Can you work these out from the model? Positions are in its coordinate system, mm. Face numbers are marked on the shaded views. Round coordinates to 2 decimals unless told otherwise and drop trailing zeros. Write each loop counter-clockwise with the first axis right and the second up, starting at its lowest first coordinate (ties: lowest second). Pieces come first, ordered by that corner, then holes. Notation, with made-up numbers: M 69.5,39 L 83.5,39 A6 ccw 83.5,50 Z; hole C 13,89 d5. An arc over 180 degrees is marked long. Answer in a Markdown table with one row per item. Add a question column.
(1) Suppose I cut it at A-A, the plane y = -40. Write out the boundary of the cut face in (x, z).
(2) I'm going to push flat-ended pins straight in: pin 1 (3.5 mm diameter, centred on x = -180.65, z = 32.92, fed in from +Y); pin 2 (12 mm diameter, centred on x = -61.5, y = 3.5, fed in from +Z); pin 3 (1 mm diameter, centred on x = -120.5, z = -0.5, fed in from -Y); pin 4 (1 mm diameter, centred on x = -169, z = 8, fed in from -Y). Where does each tip first touch, or does it pass through?
(3) If I drill on probe 1 along X at (y, z) = (-35, -1); probe 2 along X at (y, z) = (-50, -0.4); probe 3 along X at (y, z) = (76, 12), over which ranges is the centre line in solid material (lowest first)?
(4) Suppose I cut it at C-C, the plane z = 12.5. Write out the boundary of the cut face in (x, y), then the cut area to 3 significant figures.
(5) Suppose I cut it at B-B, the plane x = -92. Write out the boundary of the cut face in (y, z).
(6) If we mould it in two halves opening along Y, with no side actions, what happens to the marked faces 1 and 2? For each: released by +Y, released by -Y, zero draft, split by the parting line, or undercut.
(7) Suppose I cut it at D-D, the plane y = -15.5. Write out the boundary of the cut face in (x, z), then the cut area to 3 significant figures.
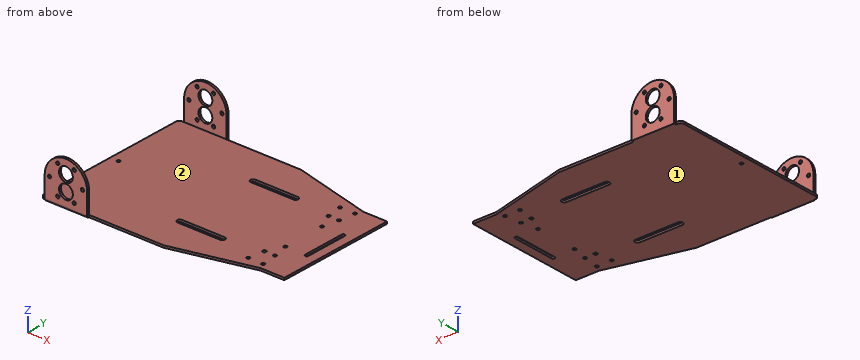
Autodesk Inventor part; units mm, degrees
ref_plane "YZ Plane" through (0, 0, 0) normal (1, 0, 0) x (0, 1, 0)
ref_plane "XZ Plane" through (0, 0, 0) normal (0, 1, 0) x (-1, 0, 0)
ref_plane "XY Plane" through (0, 0, 0) normal (0, 0, 1) x (1, 0, 0)
ref_plane "Plano de trabajo1" through (0, 0, 0) normal (0, 0, 1) x (1, 0, 0)
sketch "Boceto1" plane through (0, 0, 0) normal (0, 0, 1) x (1, 0, 0)
  line L0 (14.1, -53) -> (14.1, 53)
  line L1 (-197.9, 72) -> (-197.9, -72)
  line L2 (-194.9, -75) -> (-82.9, -75)
  line L3 (-7.9, -56) -> (14.1, -56)
  line L4 (5.6, 20) -> (5.6, -20)
  line L5 (2.6, -20) -> (2.6, 20)
  circle A0 centre (4.1, -20) radius 1.5
  circle A1 centre (4.1, 20) radius 1.5
  line L6 (-14.4, 20) -> (-14.4, -20)
  line L7 (-17.4, -20) -> (-17.4, 20)
  circle A2 centre (-15.9, -20) radius 1.5
  circle A3 centre (-15.9, 20) radius 1.5
  line L8 (-12.9, -51.5) -> (-12.9, -48.5)
  line L9 (-14.4, -36.5) -> (-14.4, -33.5)
  line L10 (-21.4, -33.5) -> (-21.4, -36.5)
  line L11 (-22.9, -48.5) -> (-22.9, -51.5)
  circle A4 centre (-24.9, -50) radius 1.5
  line L12 (-22.9, -48.5) -> (-24.9, -48.5)
  line L13 (-22.9, -51.5) -> (-24.9, -51.5)
  line L14 (-10.9, -51.5) -> (-12.9, -51.5)
  line L15 (-10.9, -48.5) -> (-12.9, -48.5)
  circle A5 centre (-10.8999, -50) radius 1.5
  line L16 (-22.9, -33.5) -> (-21.4, -33.5)
  line L17 (-22.9, -36.5) -> (-21.4, -36.5)
  circle A6 centre (-22.9, -35) radius 1.5
  line L18 (-12.9, -33.5) -> (-14.4, -33.5)
  line L19 (-12.9, -36.5) -> (-14.4, -36.5)
  circle A7 centre (-12.9, -35) radius 1.5
  line L20 (-97.9, -42.5) -> (-57.9, -42.5)
  line L21 (-57.9, -37.5) -> (-97.9, -37.5)
  circle A8 centre (-57.9, -40) radius 2.5
  circle A9 centre (-97.9, -40) radius 2.5
  line L22 (14.1, 0) -> (-197.9, 0) construction
  line L23 (-12.9, 51.5) -> (-12.9, 48.5)
  line L24 (-14.4, 36.5) -> (-14.4, 33.5)
  line L25 (-21.4, 33.5) -> (-21.4, 36.5)
  line L26 (-22.9, 48.5) -> (-22.9, 51.5)
  circle A10 centre (-24.9, 50) radius 1.5
  line L27 (-22.9, 48.5) -> (-24.9, 48.5)
  line L28 (-22.9, 51.5) -> (-24.9, 51.5)
  line L29 (-10.9, 51.5) -> (-12.9, 51.5)
  line L30 (-10.9, 48.5) -> (-12.9, 48.5)
  circle A11 centre (-10.8999, 50) radius 1.5
  line L31 (-22.9, 33.5) -> (-21.4, 33.5)
  line L32 (-22.9, 36.5) -> (-21.4, 36.5)
  circle A12 centre (-22.9, 35) radius 1.5
  line L33 (-12.9, 33.5) -> (-14.4, 33.5)
  line L34 (-12.9, 36.5) -> (-14.4, 36.5)
  circle A13 centre (-12.9, 35) radius 1.5
  line L35 (-97.9, 42.5) -> (-57.9, 42.5)
  line L36 (-57.9, 37.5) -> (-97.9, 37.5)
  circle A14 centre (-57.9, 40) radius 2.5
  circle A15 centre (-97.9, 40) radius 2.5
  line L37 (-82.8999, 75) -> (-194.9, 75)
  arc A16 (-197.9, -72) -> (-194.9, -75) centre (-194.9, -72) ccw
  arc A17 (-194.9, 75) -> (-197.9, 72) centre (-194.9, 72) ccw
  arc A18 (11.1, -56) -> (14.1, -53) centre (11.1, -53) ccw
  line L38 (-7.9, 56) -> (14.1, 56)
  arc A19 (14.1, 53) -> (11.1, 56) centre (11.1, 53) ccw
  line L39 (-7.9, -56) -> (-82.9, -75)
  line L40 (-7.9, 56) -> (-82.8999, 75)
  line L41 (-197.9, 75) -> (14.1, 75)
  line L42 (14.1, 75) -> (14.1, -75)
  line L43 (14.1, -75) -> (-197.9, -75)
  line L44 (-197.9, -75) -> (-197.9, 75)
  circle A20 centre (-189.9001, 0) radius 1.5001
  point P0 (0, 0)
  point P1 (14.1, 53)
  point P2 (-82.8999, 75)
  point P3 (-82.9, -75)
  point P4 (14.1, -53)
  point P5 (-97.8931, 37.5)
  point P6 (-97.8889, 42.5)
  point P7 (-57.9079, 42.5)
  point P8 (-57.9073, 37.5)
  point P9 (-22.8934, 36.5)
  point P10 (-21.4, 35.0152)
  point P11 (-21.4, 34.9847)
  point P12 (-22.8854, 33.5)
  point P13 (5.6, 19.9882)
  point P14 (5.6, -19.9951)
  point P15 (2.6, -19.9929)
  point P16 (2.6, 19.9946)
  point P17 (-21.4, -34.9847)
  point P18 (-21.4, -35.0152)
  point P19 (-22.8934, -36.5)
  point P20 (-22.8854, -33.5)
  point P21 (-97.8889, -42.5)
  point P22 (-97.8931, -37.5)
  point P23 (-57.9073, -37.5)
  point P24 (-57.9079, -42.5)
  dimension "d1" = 3
  dimension "d2" = 3
extrude "Extrusión1" add sketch "Boceto1" against normal blind 2 contours A18 L3 L39 L2 A16 L1 A17 L37 L40 L38 A19 L0 | L42 L3 A18 | A19 L38 L42 | L6 A2 L7 A3 | L8 L15 A5 L14 | L9 A7 L19 | L9 L18 A7 | L11 L13 A4 L12 | L29 A11 L30 L23 | L34 A13 L24 | A13 L33 L24 | L27 A10 L28 L26
ref_plane "Plano de trabajo2" through (-165.025, -77.1, 12.7883) normal (0, -1, 0) x (1, 0, 0)
sketch "Boceto2" plane through (-165.025, -77.1, 12.7883) normal (0, -1, 0) x (1, 0, 0)
  line L0 (12.125, 6.7117) -> (12.125, -14.7883)
  circle A0 centre (-0.125, 20.1351) radius 1.5
  circle A1 centre (-15.6249, 20.135) radius 1.4999
  line L1 (-1.375, 13.7117) -> (-1.375, -0.2883)
  line L2 (-27.875, -14.7883) -> (-27.875, 6.7117)
  circle A2 centre (-7.8749, 13.7117) radius 6.4999
  line L3 (-14.375, -0.2883) -> (-14.375, 13.7117)
  circle A3 centre (-7.875, -0.2883) radius 6.4999
  circle A4 centre (-23.3751, 6.7116) radius 1.5001
  circle A5 centre (-15.625, -6.7117) radius 1.5
  circle A6 centre (7.625, 6.7117) radius 1.5
  line L4 (82.125, -14.7883) -> (-29.875, -14.7883)
  line L5 (-11.348, 26.4079) -> (-4.402, 26.4079)
  circle A7 centre (-0.125, -6.7117) radius 1.5
  arc A8 (12.125, 6.7117) -> (-27.875, 6.7117) centre (-7.875, 6.4055) ccw
extrude "Extrusión2" add sketch "Boceto2" against normal up to surface (2.1 mm away) contours L0 L4 L2 A8 | L1 A3 L3 A2
fillet "Empalme1" radius 2 1 edges at (-172.9, -77.1, -2)
mirror "Simetría1" about plane through (0, 0, 0) normal (0, 1, 0) of "Extrusión2"
properties part number "Base1"
Calculated:
| question | item | result |
|---|---|---|
| 1 | outline | M -197.9,-2 L -100.4,-2 L -100.4,0 L -197.9,0 Z; M -55.4,-2 L 14.1,-2 L 14.1,0 L -55.4,0 Z |
| 2 | pin 1 | y = 77.1 |
| 2 | pin 2 | z = 0 |
| 2 | pin 3 | y = -75 |
| 2 | pin 4 | through |
| 3 | probe 1 | -197.9 to -24.4, -21.4 to -14.4, -11.4 to 14.1 |
| 3 | probe 2 | -197.9 to -26.4, -23.4 to -12.4, -9.4 to 14.1 |
| 3 | probe 3 | -192.9 to -179.38, -166.42 to -152.9 |
| 4 | outline | M -192.9,-77.1 L -179.4,-77.1 L -179.4,-75 L -192.9,-75 Z; M -192.9,75 L -179.4,75 L -179.4,77.1 L -192.9,77.1 Z; M -166.4,-77.1 L -152.9,-77.1 L -152.9,-75 L -166.4,-75 Z; M -166.4,75 L -152.9,75 L -152.9,77.1 L -166.4,77.1 Z |
| 4 | area | 113 mm² |
| 5 | outline | M -75,-2 L -42.5,-2 L -42.5,0 L -75,0 Z; M -37.5,-2 L 37.5,-2 L 37.5,0 L -37.5,0 Z; M 42.5,-2 L 75,-2 L 75,0 L 42.5,0 Z |
| 6 | face 1 | zero draft |
| 6 | face 2 | undercut |
| 7 | outline | M -197.9,-2 L 2.6,-2 L 2.6,0 L -197.9,0 Z; M 5.6,-2 L 14.1,-2 L 14.1,0 L 5.6,0 Z |
| 7 | area | 418 mm² |
